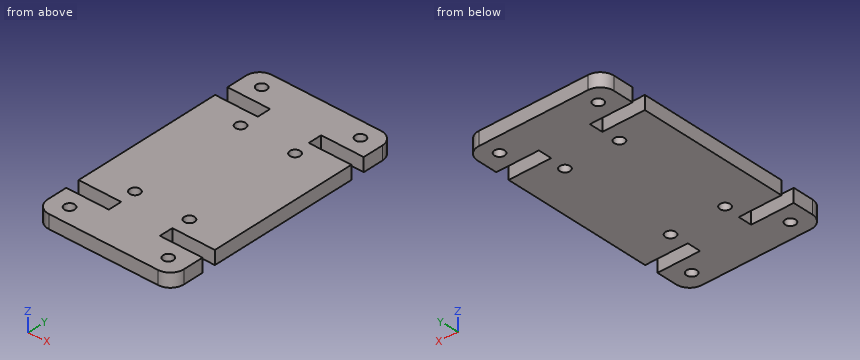
from build123d import *

# Parameters (mm, degrees)
MODEL_R             = 0.75
BOSS_EXTRUDE1_DEPTH = 2


with BuildPart() as part:
    # Model → Boss-Extrude1 (new body)
    with BuildSketch(Plane.XY):
        with BuildLine():
            Line((2, 36.1), (18, 36.1))
            ThreePointArc((18, 36.1), (19.414213562, 35.514213562), (20, 34.1))
            Line((20, 34.1), (20, 31.1))
            Line((20, 31.1), (13.75, 31.1))
            Line((13.75, 31.1), (13.75, 29.1))
            Line((13.75, 29.1), (20, 29.1))
            Line((20, 29.1), (20, 7))
            Line((20, 7), (13.75, 7))
            Line((13.75, 7), (13.75, 5))
            Line((13.75, 5), (20, 5))
            Line((20, 5), (20, 2))
            ThreePointArc((20, 2), (19.414213562, 0.585786438), (18, 0))
            Line((18, 0), (2, 0))
            ThreePointArc((2, 0), (0.585786438, 0.585786438), (0, 2))
            Line((0, 2), (0, 5))
            Line((0, 5), (6.25, 5))
            Line((6.25, 5), (6.25, 7))
            Line((6.25, 7), (0, 7))
            Line((0, 7), (0, 29.1))
            Line((0, 29.1), (6.25, 29.1))
            Line((6.25, 29.1), (6.25, 31.1))
            Line((6.25, 31.1), (0, 31.1))
            Line((0, 31.1), (0, 34.1))
            ThreePointArc((0, 34.1), (0.585786438, 35.514213562), (2, 36.1))
        make_face()
        with Locations((14, 26.6)):
            Circle(MODEL_R, mode=Mode.SUBTRACT)
        with Locations((6, 26.6)):
            Circle(MODEL_R, mode=Mode.SUBTRACT)
        with Locations((14, 9.5)):
            Circle(MODEL_R, mode=Mode.SUBTRACT)
        with Locations((6, 9.5)):
            Circle(MODEL_R, mode=Mode.SUBTRACT)
        with Locations((17.25, 2.5)):
            Circle(MODEL_R, mode=Mode.SUBTRACT)
        with Locations((2.75, 2.5)):
            Circle(MODEL_R, mode=Mode.SUBTRACT)
        with Locations((17.25, 33.6)):
            Circle(MODEL_R, mode=Mode.SUBTRACT)
        with Locations((2.75, 33.6)):
            Circle(MODEL_R, mode=Mode.SUBTRACT)
    extrude(amount=BOSS_EXTRUDE1_DEPTH)


solid = part.part
The listing builds one solid part. Answer for the finished solid, in the listing's coordinates (mm). Give positions to 0.01 mm unless a question says otherwise; leave off trailing zeros. Order: outer loops, then holes, each group sorted by start corner. A loop starts at its lowest first (then second) coordinate and runs counter-clockwise, first axis right, second up. Notation, with made-up numbers: (-9, 42) - (29, 42) arc R23 ccw to (29, 55) - close; hole circle Ø3 at (74, -24.5). An arc over 180 degrees is marked (long way). One line per item, written item: value. Start each with the question number.
1) A cutting plane is placed at B-B on y = 26.6. Give the vertices of the cut face in (x, z), then the cut area to 3 significant figures.
2) A cutting plane is placed at D-D on x = 4.25. Give the vertices of the cut face in (y, z).
3) A cutting plane is placed at C-C on z = 1.4. State how many separate pieces and enclosed holes the cut face has, then the cut area to 3 significant figures.
4) Given pin 1 Ø5 at (x, y) = (8, 13.5) entering from -Z; pin 2 Ø1 at (y, z) = (6, 1) entering from +X; pin 3 Ø1 at (y, z) = (30, 0.5) entering from -X, each flat-ended and moving along its own axis, determine where each tip first touches the part or whether it passes through.
5) Find the intervals of material crossed by L1, parallel to Y at x = 2.75, z = 1.25; L2, parallel to Y at x = 14, z = 0.9; L3, parallel to Y at x = 4, z = 0.15, in increasing order.
6) A cutting plane is placed at A-A on x = 17.25. Give the vertices of the cut face in (y, z).
Answer sheet:
1. outline: (0, 0) - (5.25, 0) - (5.25, 2) - (0, 2) - close; (6.75, 0) - (13.25, 0) - (13.25, 2) - (6.75, 2) - close; (14.75, 0) - (20, 0) - (20, 2) - (14.75, 2) - close
1. area: 34.0 mm2
2. outline: (0, 0) - (5, 0) - (5, 2) - (0, 2) - close; (7, 0) - (29.1, 0) - (29.1, 2) - (7, 2) - close; (31.1, 0) - (36.1, 0) - (36.1, 2) - (31.1, 2) - close
3. separate pieces: 1
3. enclosed holes: 8
3. area: 654 mm2
4. pin 1: stops at z = 0
4. pin 2: stops at x = 13.75
4. pin 3: stops at x = 6.25
5. L1: y = 0 to 1.75, 3.25 to 5, 7 to 29.1, 31.1 to 32.85, 34.35 to 36.1
5. L2: y = 0 to 5, 7 to 8.75, 10.25 to 25.85, 27.35 to 29.1, 31.1 to 36.1
5. L3: y = 0 to 5, 7 to 29.1, 31.1 to 36.1
6. outline: (0, 0) - (1.75, 0) - (1.75, 2) - (0, 2) - close; (3.25, 0) - (5, 0) - (5, 2) - (3.25, 2) - close; (7, 0) - (29.1, 0) - (29.1, 2) - (7, 2) - close; (31.1, 0) - (32.85, 0) - (32.85, 2) - (31.1, 2) - close; (34.35, 0) - (36.1, 0) - (36.1, 2) - (34.35, 2) - close
